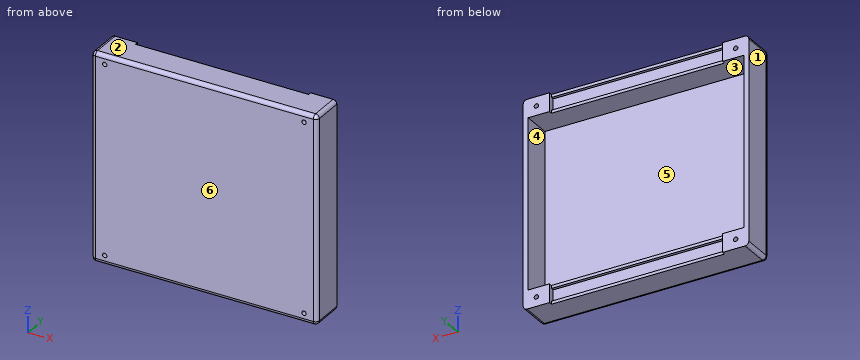
from build123d import *

# Parameters (mm, degrees)
SKETCH1_W           = 228.04
SKETCH1_H           = 209.32
BOSS_EXTRUDE1_DEPTH = 33.5
SKETCH2_W           = 218.04
SKETCH2_H           = 171.92
CUT_EXTRUDE1_DEPTH  = 28.5
SKETCH4_W           = 175
SKETCH4_H           = 18.7
CUT_EXTRUDE2_DEPTH  = 3.35
SKETCH5_W           = 175
SKETCH5_H           = 12.7
CUT_EXTRUDE3_DEPTH  = 3
SKETCH6_W           = 175
SKETCH6_H           = 18.7
CUT_EXTRUDE4_DEPTH  = 3.35
SKETCH7_W           = 175
SKETCH7_H           = 12.7
CUT_EXTRUDE5_DEPTH  = 3
SKETCH11_R          = 2.2
CUT_EXTRUDE6_DEPTH  = 33.5
FILLET3_R           = 3.81


with BuildPart() as part:
    # Sketch1 → Boss-Extrude1 (new body)
    with BuildSketch(Plane(origin=(0, 0, 0), x_dir=(1, 0, 0), z_dir=(0, 1, 0))):
        Rectangle(SKETCH1_W, SKETCH1_H)
    extrude(amount=BOSS_EXTRUDE1_DEPTH)

    # Sketch2 → Cut-Extrude1 (cut)
    with BuildSketch(Plane(origin=(0, 33.5, 0), x_dir=(1, 0, 0), z_dir=(0, 1, 0))):
        Rectangle(SKETCH2_W, SKETCH2_H)
    extrude(amount=-CUT_EXTRUDE1_DEPTH, mode=Mode.SUBTRACT)

    # Sketch4 → Cut-Extrude2 (cut)
    with BuildSketch(Plane(origin=(0, 33.5, 0), x_dir=(1, 0, 0), z_dir=(0, 1, 0))):
        with Locations((0, -95.31)):
            Rectangle(SKETCH4_W, SKETCH4_H)
    extrude(amount=-CUT_EXTRUDE2_DEPTH, mode=Mode.SUBTRACT)

    # Sketch5 → Cut-Extrude3 (cut)
    with BuildSketch(Plane(origin=(0, 30.15, 0), x_dir=(1, 0, 0), z_dir=(0, 1, 0))):
        with Locations((0, -95.31)):
            Rectangle(SKETCH5_W, SKETCH5_H)
    extrude(amount=-CUT_EXTRUDE3_DEPTH, mode=Mode.SUBTRACT)

    # Sketch6 → Cut-Extrude4 (cut)
    with BuildSketch(Plane(origin=(0, 33.5, 0), x_dir=(1, 0, 0), z_dir=(0, 1, 0))):
        with Locations((0, 95.31)):
            Rectangle(SKETCH6_W, SKETCH6_H)
    extrude(amount=-CUT_EXTRUDE4_DEPTH, mode=Mode.SUBTRACT)

    # Sketch7 → Cut-Extrude5 (cut)
    with BuildSketch(Plane(origin=(0, 30.15, 0), x_dir=(1, 0, 0), z_dir=(0, 1, 0))):
        with Locations((0, 95.31)):
            Rectangle(SKETCH7_W, SKETCH7_H)
    extrude(amount=-CUT_EXTRUDE5_DEPTH, mode=Mode.SUBTRACT)

    # Sketch11 → Cut-Extrude6 (cut)
    with BuildSketch(Plane(origin=(0, 33.5, 0), x_dir=(1, 0, 0), z_dir=(0, 1, 0))):
        with Locations(Location((100.76, 95.31, 0), (0, 0, 270))):
            Circle(SKETCH11_R)
        with Locations(Location((100.76, -95.31, 0), (0, 0, 90))):
            Circle(SKETCH11_R)
    cut_extrude6 = extrude(amount=-CUT_EXTRUDE6_DEPTH, mode=Mode.SUBTRACT)

    # Fillet3
    fillet3_edges = [part.edges().sort_by_distance(p)[0] for p in [
        (0, 0, 104.66),
        (-114.02, 0, 0),
        (0, 0, -104.66),
        (114.02, 0, 0),
        (114.02, 16.75, 104.66),
        (-114.02, 16.75, 104.66),
        (-114.02, 16.75, -104.66),
        (114.02, 16.75, -104.66),
    ]]
    fillet(fillet3_edges, radius=FILLET3_R)

    # Mirror1: Cut-Extrude6 across plane
    add(cut_extrude6.mirror(Plane.ZY), mode=Mode.SUBTRACT)


solid = part.part
Check sheet for the modelled part. Datum: model origin and axes. Units: mm. Face numbers are marked on the shaded views. A direction names the side the tool comes from. Round coordinates to 2 decimals unless told otherwise and drop trailing zeros. Loops run counter-clockwise (first coordinate to the right, second up) from the corner with the lowest first, then second, coordinate; pieces in that order, holes last.
1. Gauge pin test, flat ends, axial feed: pin 1 Ø4 at (x, z) = (2.5, -93) entering from +Y; pin 2 Ø5 at (x, z) = (39, 18) entering from -Y; pin 3 Ø0.9 at (x, z) = (-19, 88) entering from +Y. Record the tip position at first contact, or that the pin passes through.
2. Scan lines: probe 1 along X at (y, z) = (11, 95.31); probe 2 along X at (y, z) = (12, 95); probe 3 along Z at (x, y) = (-100.76, 8.5). Record each from-to range of solid material in increasing order.
3. Sectioned sample at D-D on x = 0.5. Record the boundary of the cut face in (y, z).
4. Sectioned sample at B-B on z = 65. Record the boundary of the cut face in (x, y), and give its area (3 significant figures).
5. Sectioned sample at C-C on x = 92.5. Record the boundary of the cut face in (y, z).
6. Mould release check, pull along Z, two halves, no side actions. Record for the marked faces 1, 2, 3 and 4: released by +Z, released by -Z, zero draft, split by the parting line, or undercut.
7. Set-up check for the marked faces 5 and 6: record each of +Z, -Z, +X, -X, +Y, -Y from which the full face is reachable in a straight line by a thin tool's end or side.
8. Sectioned sample at A-A on y = 16. Record the boundary of the cut face in (x, z), and give its area (3 significant figures).
Recorded:
1. pin 1: stops at y = 27.15
1. pin 2: stops at y = 0
1. pin 3: stops at y = 30.15
2. probe 1: x = -114.02 to -102.96, -98.56 to 98.56, 102.96 to 114.02
2. probe 2: x = -114.02 to -102.94, -98.58 to 98.58, 102.94 to 114.02
2. probe 3: z = -104.66 to -97.51, -93.11 to -85.96, 85.96 to 93.11, 97.51 to 104.66
3. outline: (0, -100.85) arc R3.81 ccw to (3.81, -104.66) - (30.15, -104.66) - (30.15, -101.66) - (27.15, -101.66) - (27.15, -88.96) - (30.15, -88.96) - (30.15, -85.96) - (5, -85.96) - (5, 85.96) - (30.15, 85.96) - (30.15, 88.96) - (27.15, 88.96) - (27.15, 101.66) - (30.15, 101.66) - (30.15, 104.66) - (3.81, 104.66) arc R3.81 ccw to (0, 100.85) - close
4. outline: (-114.02, 3.81) arc R3.81 ccw to (-110.21, 0) - (110.21, 0) arc R3.81 ccw to (114.02, 3.81) - (114.02, 33.5) - (109.02, 33.5) - (109.02, 5) - (-109.02, 5) - (-109.02, 33.5) - (-114.02, 33.5) - close
4. area: 1,420 mm2
5. outline: (0, -100.85) arc R3.81 ccw to (3.81, -104.66) - (33.5, -104.66) - (33.5, -85.96) - (5, -85.96) - (5, 85.96) - (33.5, 85.96) - (33.5, 104.66) - (3.81, 104.66) arc R3.81 ccw to (0, 100.85) - close
6. face 1: zero draft
6. face 2: released by +Z
6. face 3: undercut
6. face 4: undercut
7. face 5: +Y
7. face 6: +Z, -Z, +X, -X, -Y
8. outline: (-114.02, -100.85) arc R3.81 ccw to (-110.21, -104.66) - (110.21, -104.66) arc R3.81 ccw to (114.02, -100.85) - (114.02, 100.85) arc R3.81 ccw to (110.21, 104.66) - (-110.21, 104.66) arc R3.81 ccw to (-114.02, 100.85) - close; hole (-109.02, -85.96) - (109.02, -85.96) - (109.02, 85.96) - (-109.02, 85.96) - close; hole circle Ø4.4 at (-100.76, -95.31); hole circle Ø4.4 at (-100.76, 95.31); hole circle Ø4.4 at (100.76, -95.31); hole circle Ø4.4 at (100.76, 95.31)
8. area: 10,200 mm2
